Build history of the part. All positions in model axes, mm. A direction names the side the tool comes from. Round coordinates to 2 decimals unless told otherwise and drop trailing zeros. Write each loop counter-clockwise with the first axis right and the second up, starting at its lowest first coordinate (ties: lowest second). Pieces come first, ordered by that corner, then holes. Notation, with made-up numbers: (8, 11) - (51, 11) arc R20 ccw to (51, 46) - close; hole circle Ø2 at (-36.5, -23.75). An arc over 180 degrees is marked (long way). Write each question's results on one line, items separated by ' | '.
from build123d import *

# Parameters (mm, degrees)
F0_W     = 200
F0_H     = 100
F1_DEPTH = 150
F2_T     = -2.5
F3_W     = 184.218731
F3_H     = 135
F4_DEPTH = 25
F5_W     = 56.715606
F5_H     = 4.201159
F6_DEPTH = 5
F7_W     = 183.008641
F7_H     = 9.313712
F8_DEPTH = 50


with BuildPart() as f1:
    # F0 (on Top) → F1 (new body)
    with BuildSketch(Plane.XY):
        Rectangle(F0_W, F0_H)
    extrude(amount=F1_DEPTH)

    # F2
    f2_openings = [f1.faces().sort_by_distance(p)[0] for p in [
        (0, 0, 150),
    ]]
    offset(amount=F2_T, openings=f2_openings)

    # F3 (on face) → F4 (cut)
    with BuildSketch(Plane.XZ.offset(50)):
        with Locations((0.479073, 74.760462)):
            Rectangle(F3_W, F3_H)
    extrude(amount=-F4_DEPTH, mode=Mode.SUBTRACT)

    # F5 (on face) → F6 (join)
    with BuildSketch(Plane(origin=(97.5, 0, 0), x_dir=(0, -1, 0), z_dir=(-1, 0, 0))):
        with Locations((-13.760083, 93.328818)):
            Rectangle(F5_W, F5_H)
    extrude(amount=F6_DEPTH)

    # F7 (on face) → F8 (join)
    with BuildSketch(Plane.XZ.offset(-47.5)):
        with Locations((-0.239544, 145.343144)):
            Rectangle(F7_W, F7_H)
    extrude(amount=F8_DEPTH)


solid = f1.part
(1) Flat gauge pins, fed straight in: pin 1 Ø1 at (x, y) = (61, -22) entering from -Z; pin 2 Ø5 at (x, y) = (-6, -12.5) entering from +Z; pin 3 Ø1 at (x, z) = (-63, 71) entering from -Y; pin 4 Ø1.5 at (x, y) = (94, 19.5) entering from +Z. Where does each tip first touch, or does it go through?
Worked answers:
pin 1: stops at z = 0 | pin 2: stops at z = 2.5 | pin 3: stops at y = 47.5 | pin 4: stops at z = 95.43
(2) Two-plate mould, pull along Y, no slides. Class faces 5 (the flat face through (97.5, -1, 75)), 6 (the flat face through (100, -1, 74)), 7 (the flat face through (-8, -50, 147)): released by +Y, released by -Y, zero draft, split by the parting line, or undercut.
Worked answers:
face 5: undercut | face 6: zero draft | face 7: released by -Y
(3) Drill centre lines: probe 1 along X at (y, z) = (-16.5, 77.5); probe 2 along X at (y, z) = (14, 141.5); probe 3 along Z at (x, y) = (27, 23.5). Where is each one in solid material? Low to high. Write a range as [from, to].
Worked answers:
probe 1: x = [-100, -97.5], [97.5, 100] | probe 2: x = [-100, -97.5], [-91.74, 91.26], [97.5, 100] | probe 3: z = [0, 2.5], [140.69, 150]
(4) Slice it at C-C, the plane z = 132. Write the cut outline in (x, y).
Worked answers:
outline: (-100, -50) - (-91.63, -50) - (-91.63, -47.5) - (-97.5, -47.5) - (-97.5, 47.5) - (97.5, 47.5) - (97.5, -47.5) - (92.59, -47.5) - (92.59, -50) - (100, -50) - (100, 50) - (-100, 50) - close
(5) Tool access for faces 1 (the flat face through (-1, 1, 2.5)), 2 (the flat face through (92.5, 14, 93)), 3 (the flat face through (-2, 23, 140.686)), 4 (the flat face through (-2, -2.5, 145)): list every direction of +Z, -Z, +X, -X, +Y, -Y with a clear straight run to the whole face (end or side of a thin tool).
Worked answers:
face 1: none | face 2: +Z, -Y | face 3: -Y | face 4: +Z
(6) Slice it at B-B, the plane x = -17. Write the cut outline in (y, z), and give its area (3 significant figures).
Worked answers:
outline: (-50, 0) - (50, 0) - (50, 150) - (-2.5, 150) - (-2.5, 140.69) - (47.5, 140.69) - (47.5, 2.5) - (-47.5, 2.5) - (-47.5, 7.26) - (-50, 7.26) - close; (-50, 142.26) - (-47.5, 142.26) - (-47.5, 150) - (-50, 150) - close | area: 1,120 mm2
(7) Slice it at A-A, the plane y = 26. Write the cut outline in (x, z), and give its area (3 significant figures).
Worked answers:
outline: (-100, 0) - (100, 0) - (100, 150) - (97.5, 150) - (97.5, 95.43) - (92.5, 95.43) - (92.5, 91.23) - (97.5, 91.23) - (97.5, 2.5) - (-97.5, 2.5) - (-97.5, 150) - (-100, 150) - close; (-91.74, 140.69) - (91.26, 140.69) - (91.26, 150) - (-91.74, 150) - close | area: 2,960 mm2
